Input: dimensioned drawing with shaded views. Units: mm. Origin: part minimum x, y, z. A direction names the side the tool comes from. Coordinates: 2 decimals unless noted, no trailing zeros. Loops run counter-clockwise (first coordinate to the right, second up) from the corner with the lowest first, then second, coordinate; pieces in that order, holes last.
(1) Section B-B, the plane x = 84. Return loops of the section in (y, z), then the cut area to 3 significant figures.
(2) Section C-C, the plane z = 65. Return loops of the section in (x, y), then the cut area to 3 significant figures.
(3) Set-up query: the marked faces 4 and 5. Return all of +Z, -Z, +X, -X, +Y, -Y with unobstructed straight access to the full face (end or side cutting, diameter ignored); none if empty.
(4) Section A-A, the plane y = 7.75. Return loops of the section in (x, z).
(5) Contact query for flat-ended pins moving along their axis: P1, Ø1.6, axis at x = 5, z = 65, coming from the +Y side; P2, Ø2, axis at x = 68, z = 34, coming from the +Y side. Output: stop coordinate, or through.
(6) Section D-D, the plane x = 8.5. Return loops of the section in (y, z), then the cut area to 3 significant figures.
(7) Mould query, pull axis X, two halves, no side actions, for the marked faces 1, 2 and 3. Classes: released by +X, released by -X, zero draft, split by the parting line, or undercut.
(8) Line query: L1, parallel to Y at x = 69, z = 59; L2, parallel to X at y = 4.5, z = 5; L3, parallel to X at y = 9.25, z = 3. Output: solid intervals per line, ascending.
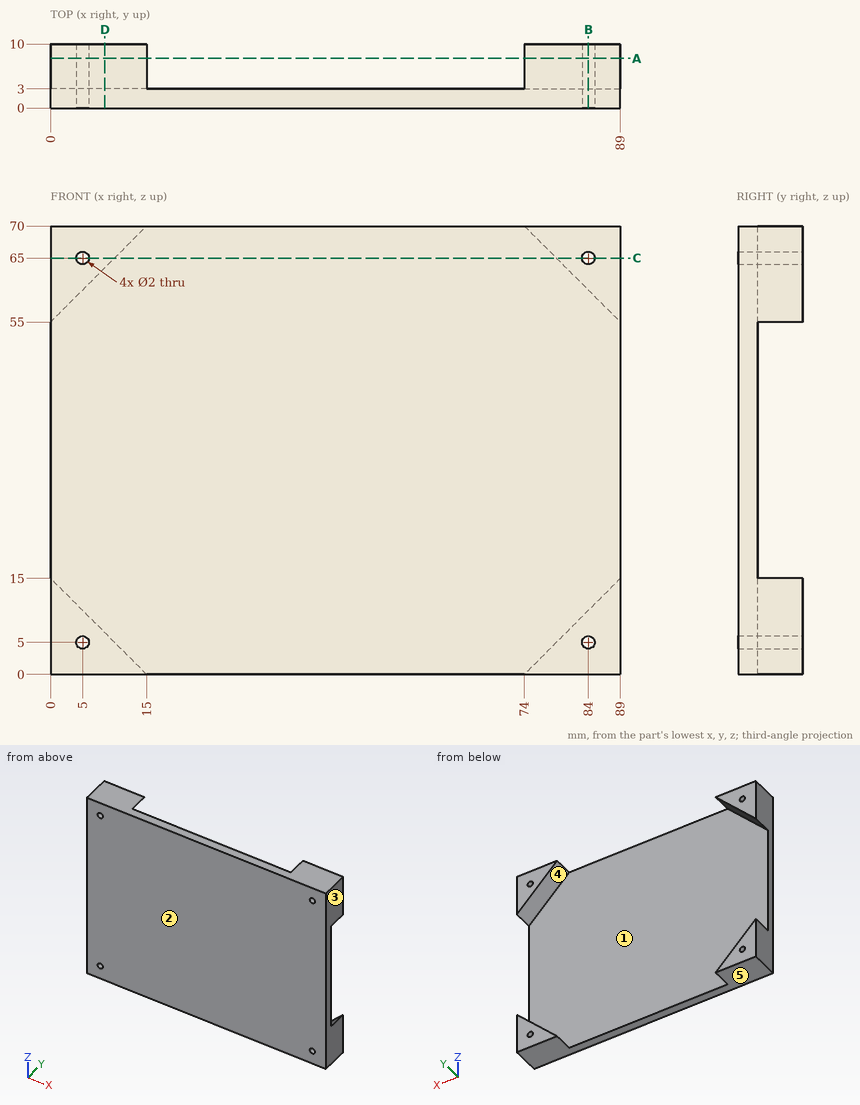
Report:
1. outline: (0, 0) - (10, 0) - (10, 4) - (0, 4) - close; (0, 6) - (10, 6) - (10, 10) - (3, 10) - (3, 60) - (10, 60) - (10, 64) - (0, 64) - close; (0, 66) - (10, 66) - (10, 70) - (0, 70) - close
1. area: 310 mm2
2. outline: (0, 0) - (4, 0) - (4, 10) - (0, 10) - close; (6, 0) - (83, 0) - (83, 10) - (79, 10) - (79, 3) - (10, 3) - (10, 10) - (6, 10) - close; (85, 0) - (89, 0) - (89, 10) - (85, 10) - close
2. area: 367 mm2
3. face 4: +Y
3. face 5: -Z, +X, -X, +Y, -Y
4. outline: (0, 0) - (15, 0) - (0, 15) - close; (0, 55) - (15, 70) - (0, 70) - close; (74, 0) - (89, 0) - (89, 15) - close; (74, 70) - (89, 55) - (89, 70) - close; hole circle Ø2 at (5, 5); hole circle Ø2 at (5, 65); hole circle Ø2 at (84, 5); hole circle Ø2 at (84, 65)
5. P1: passes through
5. P2: stops at y = 3
6. outline: (0, 0) - (10, 0) - (10, 6.5) - (3, 6.5) - (3, 63.5) - (10, 63.5) - (10, 70) - (0, 70) - close
6. area: 301 mm2
7. face 1: undercut
7. face 2: zero draft
7. face 3: released by +X
8. L1: y = 0 to 3
8. L2: x = 0 to 4, 6 to 10, 79 to 83, 85 to 89
8. L3: x = 0 to 12, 77 to 89
